Verification items for the finished model (mm, model axes). A direction names the side the tool comes from. Round coordinates to 2 decimals unless told otherwise and drop trailing zeros. Write each loop counter-clockwise with the first axis right and the second up, starting at its lowest first coordinate (ties: lowest second). Pieces come first, ordered by that corner, then holes. Notation, with made-up numbers: (12.5, 16) -> (32.5, 16) arc R15 ccw to (32.5, 34) -> close; hole circle Ø6 at (-29.5, 34.5). An arc over 180 degrees is marked (long way). Answer as a JSON object with one key per item and string values. Group by question number.
(1) Draft check along X on faces 3 (the face through (0, 1.212, -1)), 4 (the face through (1.2, -1.2, -3)), 5 (the face through (-1.45, 0.06, -10.4)). Enter one of: released by +X, released by -X, zero draft, split by the parting line, or undercut.
(2) Gauge pin test, flat ends, axial feed: pin 1 Ø1.5 at (y, z) = (-2, -5.5) entering from +X; pin 2 Ø1 at (x, y) = (2, -2) entering from -Z; pin 3 Ø3 at (y, z) = (-1, -15.5) entering from -X. Record the tip position at first contact, or that the pin passes through.
(3) Set-up check for faces 1 (the face through (1, -1, 0)), 2 (the face through (1.05, -0.61, -0.71)): record each of +Z, -Z, +X, -X, +Y, -Y from which the full face is reachable in a straight line by a thin tool's end or side.
(4) Scan lines: L1, parallel to Y at x = 0.05, z = -4; L2, parallel to Z at x = -1.85, y = 0.8; L3, parallel to Z at x = 0.15, y = 0.8. Record each from-to range of solid material in increasing order. Write a range as from..to.
(5) Sectioned sample at C-C on z = -11.75. Record the cut outline in (x, y), and give its area (3 significant figures).
(6) Sectioned sample at A-A on x = 0. Record the cut outline in (y, z) (3 decimals), and give its area (3 significant figures).
(7) Sectioned sample at D-D on y = -2.25. Record the cut outline in (x, z), and give its area (3 significant figures).
(8) Sectioned sample at B-B on y = -0.55. Record the cut outline in (x, z), and give its area (3 significant figures).
Solid Edge part; units mm, degrees
sketch "Sketch1" plane through (0, 0, 0) normal (0, 0, 1) x (1, 0, 0)
  circle A0 centre (0, 0) radius 2.725
extrude "Protrusion1" add sketch "Sketch1" against normal blind 3
sketch "Sketch2" plane through (0, 0, 0) normal (0, 0, 1) x (1, 0, 0)
  line L0 (-0.7, -1.2124) -> (-1.05, -0.6062)
  line L1 (-1.4, 0) -> (-1.05, -0.6062)
  line L2 (-1.4, 0) -> (-1.05, 0.6062)
  line L3 (-0.7, 1.2124) -> (-1.05, 0.6062)
  line L4 (-0.7, 1.2124) -> (0, 1.2124)
  line L5 (0.7, 1.2124) -> (0, 1.2124)
  line L6 (0.7, 1.2124) -> (1.05, 0.6062)
  line L7 (1.4, 0) -> (1.05, 0.6062)
  line L8 (1.4, 0) -> (1.05, -0.6062)
  line L9 (0.7, -1.2124) -> (1.05, -0.6062)
  line L10 (0.7, -1.2124) -> (0, -1.2124)
  line L11 (-0.7, -1.2124) -> (0, -1.2124)
extrude "ExtrudedCutout_1" cut sketch "Sketch2" against normal blind 1.45
sketch "Sketch3" plane through (0, 0, -3) normal (0, 0, -1) x (1, 0, 0)
  circle A0 centre (0, 0) radius 1.45
extrude "ExtrudedProtrusion_2" add sketch "Sketch3" along normal blind 15
Computed values:
{
 "1": {"face 3": "undercut", "face 4": "zero draft", "face 5": "split by the parting line"},
 "2": {"pin 1": "x = 0.73", "pin 2": "z = -3", "pin 3": "x = -1.45"},
 "3": {"face 1": "+Z, +X, -X, +Y, -Y", "face 2": "+Z"},
 "4": {"L1": "-1.45..1.45", "L2": "-3..0", "L3": "-18..-1.45"},
 "5": {"outline": "circle Ø2.9 at (0, 0)", "area": "6.61 mm2"},
 "6": {"outline": "(-2.725, -3) -> (-1.45, -3) -> (-1.45, -18) -> (1.45, -18) -> (1.45, -3) -> (2.725, -3) -> (2.725, 0) -> (1.212, 0) -> (1.212, -1.45) -> (-1.212, -1.45) -> (-1.212, 0) -> (-2.725, 0) -> close", "area": "56.3 mm2"},
 "7": {"outline": "(-1.54, -3) -> (1.54, -3) -> (1.54, 0) -> (-1.54, 0) -> close", "area": "9.22 mm2"},
 "8": {"outline": "(-2.67, -3) -> (-1.34, -3) -> (-1.34, -18) -> (1.34, -18) -> (1.34, -3) -> (2.67, -3) -> (2.67, 0) -> (1.08, 0) -> (1.08, -1.45) -> (-1.08, -1.45) -> (-1.08, 0) -> (-2.67, 0) -> close", "area": "53.1 mm2"}
}
